Here's the drawing with two shaded views (mm, measured from the low corner). I have some questions. Give positions to 0.01 mm unless a question says otherwise; leave off trailing zeros. Write each loop counter-clockwise with the first axis right and the second up, starting at its lowest first coordinate (ties: lowest second). Pieces come first, ordered by that corner, then holes. Notation, with made-up numbers: M 72.5,-35.75 L 76.5,-35.75 A21 ccw 76.5,-24.75 Z; hole C 87,51.5 d6. An arc over 180 degrees is marked long. Use one line per item in the form item = value. Start each with the question number.
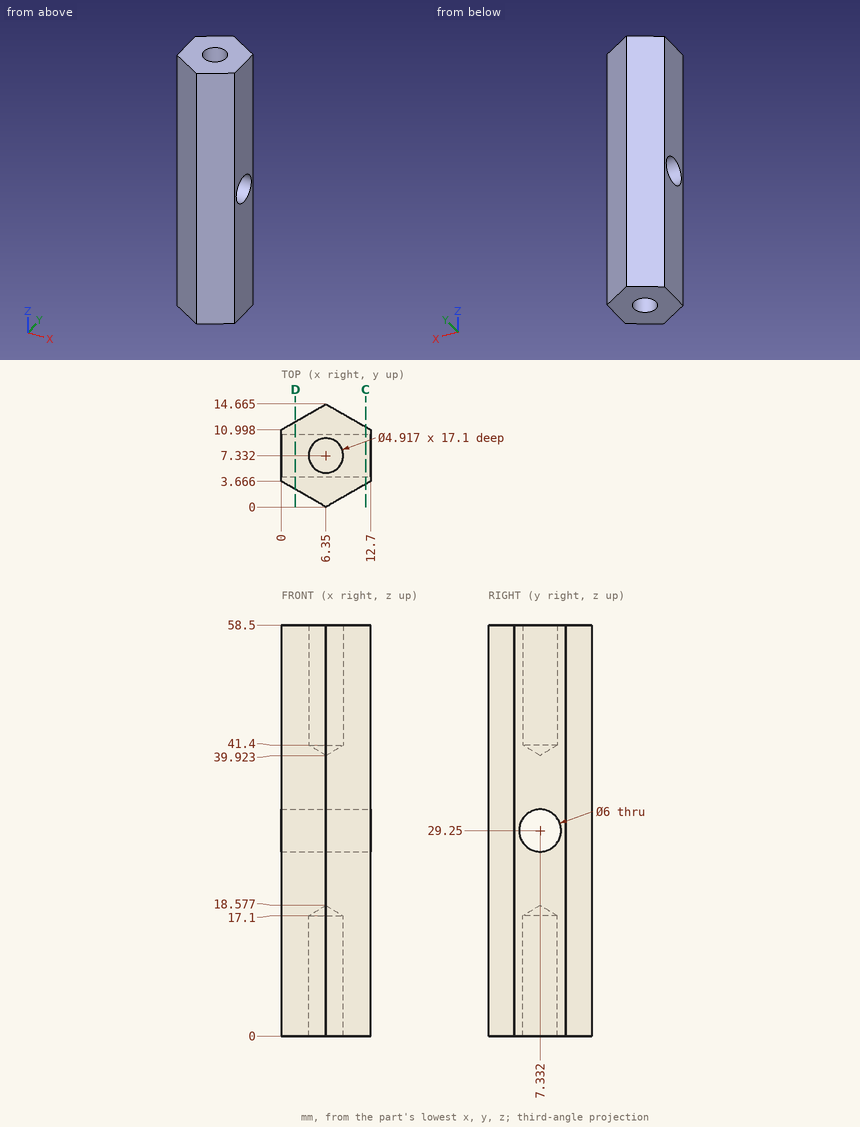
1) Suppose I cut it at D-D, the plane x = 2. List the corners of the cut face in (y, z) for me, and give its area (3 significant figures).
2) Will these pins go through, and if not, where does the flat tip stop? P1, Ø1.5, axis at y = 2.5, z = 15.5, coming from the +X side; P2, Ø1, axis at y = 12.5, z = 47.5, coming from the +X side (1 decimal); P3, Ø1.5, axis at y = 8.5, z = 30, coming from the -X side; P4, Ø3, axis at x = 6.35, y = 7.33, coming from the +Z side (1 decimal).
3) Suppose I cut it at C-C, the plane x = 12. List the corners of the cut face in (y, z) for me.
4) Please list where these lines run through material, in increasing order: line 1 (Y direction, x = 5.5, z = 29.25) (1 decimal); line 2 (Z direction, x = 1.25, y = 6.25); line 3 (Z direction, x = 3.5, y = 9.75) (1 decimal).
Checks:
q1.outline = M 2.51,0 L 12.15,0 L 12.15,58.5 L 2.51,58.5 Z; hole C 7.33,29.25 d6
q1.area = 536 mm^2
q2.P1 = 11.98
q2.P2 = 11
q2.P3 = through
q2.P4 = 40.8
q3.outline = M 3.26,0 L 11.4,0 L 11.4,58.5 L 3.26,58.5 Z; hole C 7.33,29.25 d6
q4.line_1 = 0.5 to 4.3, 10.3 to 14.2
q4.line_2 = 0 to 26.45, 32.05 to 58.5
q4.line_3 = 0 to 27.5, 31 to 58.5
